```python
from build123d import *

# Parameters (mm, degrees)
SKETCH_2_R          = 10
EXTRUDE_1_DEPTH     = 65
CUT_EXTRUDE_2_DEPTH = 5
CUT_EXTRUDE_3_DEPTH = 5


with BuildPart() as part:
    # 草图2 → 凸台-拉伸1 (new body)
    with BuildSketch(Plane(origin=(0, 10, 0), x_dir=(1, 0, 0), z_dir=(0, 1, 0))):
        Circle(SKETCH_2_R)
    extrude(amount=EXTRUDE_1_DEPTH)

    # 草图5 → 切除-拉伸2 (cut)
    with BuildSketch(Plane.XY.offset(10)):
        with BuildLine():
            Line((4.341808906, 40.859733082), (4.341808906, 25.456649106))
            ThreePointArc((4.341808906, 25.456649106), (0, 21.114840199), (-4.341808906, 25.456649106))
            Line((-4.341808906, 25.456649106), (-4.341808906, 40.859733082))
            ThreePointArc((-4.341808906, 40.859733082), (0, 45.201541988), (4.341808906, 40.859733082))
        make_face()
    extrude(amount=-CUT_EXTRUDE_2_DEPTH, mode=Mode.SUBTRACT)

    # 草图6 → 切除-拉伸3 (cut)
    with BuildSketch(Plane.XY.offset(10)):
        with BuildLine():
            Line((3.451393492, 67.868636429), (3.451393492, 53.092358039))
            ThreePointArc((3.451393492, 53.092358039), (0, 49.640964547), (-3.451393492, 53.092358039))
            Line((-3.451393492, 53.092358039), (-3.451393492, 67.868636429))
            ThreePointArc((-3.451393492, 67.868636429), (0, 71.320029921), (3.451393492, 67.868636429))
        make_face()
    extrude(amount=-CUT_EXTRUDE_3_DEPTH, mode=Mode.SUBTRACT)


solid = part.part
```
Build history of the part. All positions in model axes, mm. A direction names the side the tool comes from. Round coordinates to 2 decimals unless told otherwise and drop trailing zeros. Write each loop counter-clockwise with the first axis right and the second up, starting at its lowest first coordinate (ties: lowest second). Pieces come first, ordered by that corner, then holes. Notation, with made-up numbers: (11.25, -8) - (55.25, -8) arc R21 cw to (55.25, 18) - close; hole circle Ø8 at (66, -30.5). An arc over 180 degrees is marked (long way). Write each question's results on one line, items separated by ' | '. Start each with the question number.
Item 1: Which spindle directions (+Z, -Z, +X, -X, +Y, -Y) get a long thin tool onto all of the face, cutting with end or side? Do faces 1 (the face through (5.38, 42.04, -8.43)), 2 (the face through (4.342, 33, 7)). Say none if no direction does.
Item 2: Saw through at C-C (y = 65.5). Write the cut outline in (x, z), and give its area (3 significant figures).
Item 3: Drop flat-ended pins along their axis: P1, Ø3, axis at y = 32.5, z = 6, coming from the +X side; P2, Ø6, axis at y = 63.5, z = -6.5, coming from the +X side; P3, Ø1.3, axis at y = 59.5, z = 8, coming from the +X side. Give the stop position or say it passes through.
Item 4: Saw through at A-A (x = 0). Write the cut outline in (y, z).
Item 5: Wall check: L1, parallel to Y at x = -4, z = 5.75; L2, parallel to Z at x = 0.25, y = 15; L3, parallel to Y at x = 2.25, z = 6. Give the ranges that are in metal, low to high. Write a range as [from, to].
Item 6: Mould opens along Y. For faces 3 (the face through (0, 75, 0)), 4 (the face through (0, 61, 5)), 5 (the face through (0, 10, 0)) say: pulls with the +Y half, pulls with the -Y half, needs draft (parallel to the pull), parting line crosses it, or undercut.
Item 7: Saw through at B-B (z = -6). Write the cut outline in (x, y).
Results are:
1) face 1: +Y, -Y | face 2: +Z
2) outline: (-3.45, 5) - (-3.45, 9.39) arc R10 ccw (long way) to (3.45, 9.39) - (3.45, 5) - close | area: 281 mm²
3) P1: stops at x = 8.93 | P2: stops at x = 9.37 | P3: stops at x = 6.78
4) outline: (10, -10) - (75, -10) - (75, 10) - (71.32, 10) - (71.32, 5) - (49.64, 5) - (49.64, 10) - (45.2, 10) - (45.2, 5) - (21.11, 5) - (21.11, 10) - (10, 10) - close
5) L1: y = [10, 23.77], [42.55, 75] | L2: z = [-10, 10] | L3: y = [10, 21.74], [44.57, 50.48], [70.49, 75]
6) face 3: pulls with the +Y half | face 4: undercut | face 5: pulls with the -Y half
7) outline: (-8, 10) - (8, 10) - (8, 75) - (-8, 75) - close
